Can you work these out from the model? Positions are in its coordinate system, mm. A direction names the side the tool comes from. Coordinates: 2 decimals unless noted, no trailing zeros. Order: outer loops, then holes, each group sorted by start corner. A loop starts at its lowest first (then second) coordinate and runs counter-clockwise, first axis right, second up. Notation, with made-up numbers: (83, 50.5) -> (102, 50.5) arc R15 ccw to (102, 68.5) -> close; hole circle Ø3 at (67.5, -22.75). An arc over 180 degrees is marked (long way). Answer in a Markdown table with one row per item.
```python
from build123d import *

# Parameters (mm, degrees)
BOSS_EXTRUDE1_DEPTH             = 5
SKETCH4_R                       = 7.5
BOSS_EXTRUDE3_DEPTH             = 8.75
SKETCH5_R                       = 2.5
CUT_EXTRUDE2_DEPTH              = 10
CBORE_FOR_M5_SBHCS1_D           = 5.5
CBORE_FOR_M5_SBHCS1_CBORE_D     = 10.5
CBORE_FOR_M5_SBHCS1_CBORE_DEPTH = 2.75
SKETCH8_R                       = 2.5
CUT_EXTRUDE3_DEPTH              = 10
CHAMFER1_SIZE                   = 1


with BuildPart() as part:
    # Sketch2 → Boss-Extrude1 (new body)
    with BuildSketch(Plane.XY):
        with BuildLine():
            Line((-37.5, 12), (37.5, 12))
            ThreePointArc((37.5, 12), (49.5, 0), (37.5, -12))
            Line((37.5, -12), (-37.5, -12))
            ThreePointArc((-37.5, -12), (-49.5, 0), (-37.5, 12))
        make_face()
    extrude(amount=BOSS_EXTRUDE1_DEPTH)

    # Sketch4 → Boss-Extrude3 (add)
    with BuildSketch(Plane.XY):
        Circle(SKETCH4_R)
    extrude(amount=BOSS_EXTRUDE3_DEPTH)

    # Sketch5 → Cut-Extrude2 (cut)
    with BuildSketch(Plane.XY.offset(8.75)):
        Circle(SKETCH5_R)
    extrude(amount=-CUT_EXTRUDE2_DEPTH, mode=Mode.SUBTRACT)

    # CBORE for M5 SBHCS1 (through all)
    with Locations(Plane.XY.offset(5)):
        with Locations((-37.5, 0)):
            CounterBoreHole(CBORE_FOR_M5_SBHCS1_D / 2, CBORE_FOR_M5_SBHCS1_CBORE_D / 2, CBORE_FOR_M5_SBHCS1_CBORE_DEPTH)

    # Sketch8 → Cut-Extrude3 (cut)
    with BuildSketch(Plane.XY.offset(5)):
        with Locations((37.5, 0)):
            Circle(SKETCH8_R)
    extrude(amount=-CUT_EXTRUDE3_DEPTH, mode=Mode.SUBTRACT)

    # Chamfer1
    chamfer1_edges = [part.edges().sort_by_distance(p)[0] for p in [
        (49.5, 0, 5),
        (-7.5, 0, 8.75),
        (0, 12, 5),
        (-49.5, 0, 5),
        (0, 12, 0),
        (49.5, 0, 0),
        (0, -12, 0),
        (-49.5, 0, 0),
        (0, -12, 5),
    ]]
    chamfer(chamfer1_edges, length=CHAMFER1_SIZE)


solid = part.part
```
(1) Suppose I cut it at A-A (x = 0). Please give me the cut outline in (y, z), and give its area (4 significant figures).
Response values:
| item | result |
|---|---|
| outline | (-12, 1) -> (-11, 0) -> (-2.5, 0) -> (-2.5, 8.75) -> (-6.5, 8.75) -> (-7.5, 7.75) -> (-7.5, 5) -> (-11, 5) -> (-12, 4) -> close; (2.5, 0) -> (11, 0) -> (12, 1) -> (12, 4) -> (11, 5) -> (7.5, 5) -> (7.5, 7.75) -> (6.5, 8.75) -> (2.5, 8.75) -> close |
| area | 129.5 mm2 |
(2) We'd pull the mould along X, two halves only. Please class faces 3 (the conical face through (-48.7, -0.2, 0.2)), 4 (the cylindrical face through (-34.753, 0.121, 1.109)), 5 (the conical face through (48.7, 0.2, 0.2)): +X half, -X half, draft (parallel to the pull), parting line (faces both ways), or undercut.
Response values:
| item | result |
|---|---|
| face 3 | -X half |
| face 4 | undercut |
| face 5 | +X half |
(3) Will these pins go through, and if not, where does the flat tip stop? pin 1 Ø3.5 at (x, y) = (-37.5, 0) entering from -Z; pin 2 Ø6 at (x, y) = (37.5, 0) entering from +Z; pin 3 Ø9.5 at (x, y) = (-37.5, 0) entering from +Z; pin 4 Ø3 at (y, z) = (-8.5, 5) entering from +X.
Response values:
| item | result |
|---|---|
| pin 1 | through |
| pin 2 | z = 5 |
| pin 3 | z = 2.25 |
| pin 4 | x = 46.96 |
(4) Suppose I cut it at C-C (x = -19.5). Please give me the cut outline in (y, z), and give its area (3 significant figures).
Response values:
| item | result |
|---|---|
| outline | (-12, 1) -> (-11, 0) -> (11, 0) -> (12, 1) -> (12, 4) -> (11, 5) -> (-11, 5) -> (-12, 4) -> close |
| area | 118 mm2 |
(5) On a 3-axis mill with a long thin cutter (end or side, diameter ignored), from which of +Z, -Z, +X, -X, +Y, -Y can I reach the whole of each face in a straight line? I mean faces 1 (the flat face through (-35, -2, 2.25)), 2 (the cylindrical face through (39.81, -0.96, 2.54)). Say none if no direction works.
Response values:
| item | result |
|---|---|
| face 1 | +Z |
| face 2 | +Z, -Z |
(6) Suppose I cut it at B-B (y = 0). Count the separate pieces of the cut face and the enclosed holes in it, and give its area (3 significant figures).
Response values:
| item | result |
|---|---|
| separate pieces | 4 |
| enclosed holes | 0 |
| area | 438 mm2 |
(7) I need wall thicknesses on line 1 (X direction, y = 2, z = 0.75); line 2 (Z direction, x = -10, y = 2.25); line 3 (Y direction, x = 37.5, z = 2.7). Which ranges of each line are inside material? Lowest first, please. Write a range as [from, to].
Response values:
| item | result |
|---|---|
| line 1 | [-49.08, -39.39], [-35.61, -1.5], [1.5, 36], [39, 49.08] |
| line 2 | [0, 5] |
| line 3 | [-12, -2.5], [2.5, 12] |
